The listing builds one solid part. Answer for the finished solid, in the listing's coordinates (mm). A direction names the side the tool comes from. Coordinates: 2 decimals unless noted, no trailing zeros. Order: outer loops, then holes, each group sorted by start corner. A loop starts at its lowest first (then second) coordinate and runs counter-clockwise, first axis right, second up. Notation, with made-up numbers: (73.5, 47) - (126.5, 47) arc R35 ccw to (126.5, 81) - close; hole circle Ø3 at (82.5, -10). An arc over 180 degrees is marked (long way). One line per item, written item: value. Start each with the question number.
```python
from build123d import *

# Parameters (mm, degrees)
SKETCH2_W           = 23.651183611
SKETCH2_H           = 19.920292675
SKETCH2_W_2         = 19.320685203
SKETCH2_H_2         = 26.582597918
SKETCH2_W_3         = 22
SKETCH2_H_3         = 18.920946888
BOSS_EXTRUDE1_DEPTH = 14


with BuildPart() as part:
    # Sketch2 → Boss-Extrude1 (new body)
    with BuildSketch(Plane(origin=(0, 0, 0), x_dir=(1, 0, 0), z_dir=(0, 1, 0))):
        Polygon((-27.908593219, 57.483539187), (-27.908593219, -57.424852572), (-0.405302454, -57.424852572), (-0.405302454, -19.455651499), (28.437596205, -19.455651499), (28.437596205, -13.887867334), (0.143608651, -13.887867334), (0.143608651, 0.105967325), (28.472121021, 0.105967325), (28.472121021, 5.282539019), (-0.501944112, 5.282539019), (-0.501944112, 19.945920068), (28.807431377, 19.945920068), (28.807431377, 24.716415232), (0, 24.716415232), (0, 57.483539187), align=None)
        with Locations((-13.80552661, 36.856875137)):
            Rectangle(SKETCH2_W, SKETCH2_H, mode=Mode.SUBTRACT)
        with Locations((-13.172607612, 3.945087239)):
            Rectangle(SKETCH2_W_2, SKETCH2_H_2, mode=Mode.SUBTRACT)
        with Locations((-13.207270194, -39.259962259)):
            Rectangle(SKETCH2_W_3, SKETCH2_H_3, mode=Mode.SUBTRACT)
    extrude(amount=BOSS_EXTRUDE1_DEPTH)


solid = part.part
```
(1) Consider probe 1 along Z at (x, y) = (4, 6); probe 2 along Z at (x, y) = (-20, 11); probe 3 along X at (y, z) = (13.25, 33). Determine where each line is inside the solid, lowest interval first.
(2) The part is cut by section D-D on z = 37. Determine the outline of the cut face in (x, y).
(3) Flat-ended cylindrical pins translate along their axes: pin 1 Ø1 at (y, z) = (11, 44.5) entering from +X; pin 2 Ø7 at (y, z) = (5.5, -15.5) entering from +X; pin 3 Ø1 at (x, z) = (9.5, 21) entering from +Y; pin 4 Ø7 at (x, y) = (19, 4.5) entering from +Z. Find the tip coordinate at first contact, or state that the pin passes through.
(4) For a pull along Z with two mould halves and no side action, classify faces 1 (the face through (-2, 0, -5)), 2 (the face through (15, 7, -24.716)), 3 (the face through (14, 7, 19.456)), 4 (the face through (14, 7, -19.946)) as pulls with the +Z half, pulls with the -Z half, needs draft (parallel to the pull), parting line crosses it, or undercut.
(5) The part is cut by section A-A on z = -43.5. Determine the outline of the cut face in (x, y).
(6) The part is cut by section B-B on x = -16. Determine the outline of the cut face in (y, z).
(7) The part is cut by section C-C on y = 9. Determine the outline of the cut face in (x, z).
(8) For faces 5 (the face through (14, 7, -5.283)), 6 (the face through (-13, 7, 9.346)), 7 (the face through (28.438, 7, 17)), 8 (the face through (-2, 14, -5)), 9 (the face through (0, 7, -41)), determine the directions among +Z, -Z, +X, -X, +Y, -Y from which every point of the face is accessible in a straight line to the end or side of a thin tool.
Completed:
1. probe 1: z = -24.72 to -19.95, -5.28 to -0.11, 13.89 to 19.46
1. probe 2: z = -57.48 to -46.82, -26.9 to -17.24, 9.35 to 29.8, 48.72 to 57.42
1. probe 3: x = -27.91 to -24.21, -2.21 to -0.41
2. outline: (-27.91, 0) - (-24.21, 0) - (-24.21, 14) - (-27.91, 14) - close; (-2.21, 0) - (-0.41, 0) - (-0.41, 14) - (-2.21, 14) - close
3. pin 1: stops at x = -0.41
3. pin 2: stops at x = -0.5
3. pin 3: passes through
3. pin 4: stops at z = 19.46
4. face 1: needs draft
4. face 2: pulls with the -Z half
4. face 3: pulls with the +Z half
4. face 4: undercut
5. outline: (-27.91, 0) - (-25.63, 0) - (-25.63, 14) - (-27.91, 14) - close; (-1.98, 0) - (0, 0) - (0, 14) - (-1.98, 14) - close
6. outline: (0, -57.48) - (14, -57.48) - (14, -46.82) - (0, -46.82) - close; (0, -26.9) - (14, -26.9) - (14, -17.24) - (0, -17.24) - close; (0, 9.35) - (14, 9.35) - (14, 29.8) - (0, 29.8) - close; (0, 48.72) - (14, 48.72) - (14, 57.42) - (0, 57.42) - close
7. outline: (-27.91, -57.48) - (0, -57.48) - (0, -24.72) - (28.81, -24.72) - (28.81, -19.95) - (-0.5, -19.95) - (-0.5, -5.28) - (28.47, -5.28) - (28.47, -0.11) - (0.14, -0.11) - (0.14, 13.89) - (28.44, 13.89) - (28.44, 19.46) - (-0.41, 19.46) - (-0.41, 57.42) - (-27.91, 57.42) - close; hole (-25.63, -46.82) - (-1.98, -46.82) - (-1.98, -26.9) - (-25.63, -26.9) - close; hole (-24.21, 29.8) - (-2.21, 29.8) - (-2.21, 48.72) - (-24.21, 48.72) - close; hole (-22.83, -17.24) - (-3.51, -17.24) - (-3.51, 9.35) - (-22.83, 9.35) - close
8. face 5: +X, +Y, -Y
8. face 6: +Y, -Y
8. face 7: +Z, +X, +Y, -Y
8. face 8: +Z, -Z, +X, -X, +Y
8. face 9: -Z, +X, +Y, -Y
